```python
from build123d import *

# Parameters (mm, degrees)
F0_R     = 12.7
F1_DEPTH = 25.4
F3_DEPTH = 25.4
F4_R     = 12.7


with BuildPart() as f1:
    # F0 (on Front) → F1 (new body)
    with BuildSketch(Plane.XZ):
        with BuildLine():
            Line((44.0387030303, 9.6043962192), (-43.3234238415, 68.7387245609))
            ThreePointArc((-43.3234238415, 68.7387245609), (-69.4675563013, 70.1409955321), (-82.9612969697, 47.7043962192))
            Line((-82.9612969697, 47.7043962192), (-82.9612969697, -3.0956037808))
            Line((-82.9612969697, -3.0956037808), (44.0387030303, -3.0956037808))
            Line((44.0387030303, -3.0956037808), (44.0387030303, 9.6043962192))
        make_face()
        with Locations((-57.5612969697, 47.7043962192)):
            Circle(F0_R, mode=Mode.SUBTRACT)
    extrude(amount=F1_DEPTH)

    # F2 (on face) → F3 (join)
    with BuildSketch(Plane.XZ.offset(25.4)):
        with BuildLine():
            Line((44.0387030303, -3.0956037808), (44.0387030303, 9.6043962192))
            Line((44.0387030303, 9.6043962192), (-32.1612969697, 10.3719634618))
            Line((-32.1612969697, 10.3719634618), (-32.1612969697, 47.7043962192))
            ThreePointArc((-32.1612969697, 47.7043962192), (-35.1246976568, 59.6106555508), (-43.3234238415, 68.7387245609))
            ThreePointArc((-43.3234238415, 68.7387245609), (-69.4675563013, 70.1409955321), (-82.9612969697, 47.7043962192))
            Line((-82.9612969697, 47.7043962192), (-82.9612969697, -3.0956037808))
            Line((-82.9612969697, -3.0956037808), (44.0387030303, -3.0956037808))
        make_face()
        with BuildLine():
            ThreePointArc((-70.2612969697, 47.7043962192), (-57.5612969697, 60.4043962192), (-44.8612969697, 47.7043962192))
            ThreePointArc((-44.8612969697, 47.7043962192), (-57.5612969697, 35.0043962192), (-70.2612969697, 47.7043962192))
        make_face(mode=Mode.SUBTRACT)
    extrude(amount=F3_DEPTH)

    # F4
    f4_edges = [f1.edges().sort_by_distance(p)[0] for p in [
        (44.038703, -50.8, 3.254396),
    ]]
    fillet(f4_edges, radius=F4_R)


solid = f1.part
```
Work out the finished part from the listing and answer in its coordinate system (mm). A direction names the side the tool comes from. Round coordinates to 2 decimals unless told otherwise and drop trailing zeros. Loops run counter-clockwise (first coordinate to the right, second up) from the corner with the lowest first, then second, coordinate; pieces in that order, holes last.
(1) For faces 1 (the flat face through (-6, -25.4, 28)), 2 (the flat face through (-82.961, -25, 23)), determine the directions among +Z, -Z, +X, -X, +Y, -Y from which every point of the face is accessible in a straight line to the end or side of a thin tool.
Computed values:
face 1: +Z, +X, -Y
face 2: +Z, -Z, -X, +Y, -Y
(2) The part is cut by section D-D, the plane y = -19. Give the vertices of the cut face in (x, z), and give its area (3 significant figures).
Computed values:
outline: (-82.96, -3.1) - (44.04, -3.1) - (44.04, 9.6) - (-43.32, 68.74) arc R25.4 ccw to (-82.96, 47.7) - close; hole circle Ø25.4 at (-57.56, 47.7)
area: 6,050 mm2
(3) The mould has two halves that part along Z. Classify faces 3 (the cylindrical face through (-70.25, -25.04, 47.15)), 4 (the flat face through (44.039, -19, 3)), 5 (the flat face through (0.969, -12.522, 38.758)): pulls with the +Z half, pulls with the -Z half, needs draft (parallel to the pull), parting line crosses it, or undercut.
Computed values:
face 3: undercut
face 4: needs draft
face 5: pulls with the +Z half
(4) The part is cut by section A-A, the plane y = -29. Give the vertices of the cut face in (x, z), and give its area (3 significant figures).
Computed values:
outline: (-82.96, -3.1) - (44.04, -3.1) - (44.04, 9.6) - (-32.16, 10.37) - (-32.16, 47.7) arc R25.4 ccw to (-82.96, 47.7) - close; hole circle Ø25.4 at (-57.56, 47.7)
area: 4,080 mm2
(5) The part is cut by section B-B, the plane z = 58.5. Give the vertices of the cut face in (x, y), and give its area (3 significant figures).
Computed values:
outline: (-80.55, -50.8) - (-64.25, -50.8) - (-64.25, 0) - (-80.55, 0) - close; (-50.87, -50.8) - (-34.57, -50.8) - (-34.57, -25.4) - (-28.2, -25.4) - (-28.2, 0) - (-50.87, 0) - close
area: 1,820 mm2
(6) The part is cut by section C-C, the plane x = -55.5. Give the vertices of the cut face in (y, z), and give its area (3 significant figures).
Computed values:
outline: (-50.8, -3.1) - (0, -3.1) - (0, 35.17) - (-50.8, 35.17) - close; (-50.8, 60.24) - (0, 60.24) - (0, 73.02) - (-50.8, 73.02) - close
area: 2,590 mm2
(7) Find the intervals of material crossed by L1, parallel to X at y = -48.5, z = 47; L2, parallel to X at y = -20.5, z = 53.5; L3, parallel to Z at x = -69, y = -33.5, in increasing order.
Computed values:
L1: x = -82.96 to -70.24, -44.88 to -32.16
L2: x = -82.29 to -68.86, -46.26 to -20.81
L3: z = -3.1 to 42.19, 53.22 to 70.38
(8) Each of these flat-tipped pins is pushed along its axis until it touches: P1, Ø4, axis at y = -41.5, z = 65, coming from the +X side; P2, Ø8, axis at y = -40, z = 53, coming from the +X side; P3, Ø2, axis at x = -14, y = -5.5, coming from the +Z side; P4, Ø23, axis at x = -57.56, z = 47.7, coming from the -Y side. Where does it stop, or does it pass through?
Computed values:
P1: stops at x = -37.28
P2: stops at x = -32.19
P3: stops at z = 49.57
P4: passes through
